```python
from build123d import *

# Parameters (mm, degrees)
CYLINDER002_R       = 0.3
CYLINDER002_DEPTH   = 10
CYLINDER001_R       = 0.3
CYLINDER001_DEPTH   = 10
CYLINDER_R          = 5.75
CYLINDER_DEPTH      = 6
CYLINDER_ROLL_ANGLE = 90
FILLET_R            = 2.2


with BuildPart() as pin002:
    # Cylinder002 → Cylinder002 (new body)
    with BuildSketch(Plane(origin=(2.5, 0, -3), x_dir=(1, 0, 0), z_dir=(0, 0, 1))):
        Circle(CYLINDER002_R)
    extrude(amount=CYLINDER002_DEPTH)


with BuildPart() as pin1:
    # Cylinder001 → Cylinder001 (new body)
    with BuildSketch(Plane(origin=(-2.5, 0, -3), x_dir=(1, 0, 0), z_dir=(0, 0, 1))):
        Circle(CYLINDER001_R)
    extrude(amount=CYLINDER001_DEPTH)


with BuildPart() as obj1:
    # Cylinder → Cylinder (new body)
    with BuildSketch(Plane.XY):
        Circle(CYLINDER_R)
    extrude(amount=CYLINDER_DEPTH)


with BuildPart() as obj1_1:
    # Cylinder roll: moved
    add(obj1.part.rotate(Axis((0, 0, 0), (1, 0, 0)), CYLINDER_ROLL_ANGLE))


with BuildPart() as obj1_2:
    # Cylinder placement: moved
    add(obj1_1.part.moved(Location((0, 3, 10.25))))

    # Fillet
    fillet_edges = [obj1_2.edges().sort_by_distance(p)[0] for p in [
        (-5.75, -3, 10.25),
        (-5.75, 3, 10.25),
    ]]
    fillet(fillet_edges, radius=FILLET_R)

    # Fusion: union pin002, pin1
    add(pin002.part)
    add(pin1.part)


solid = obj1_2.part
```
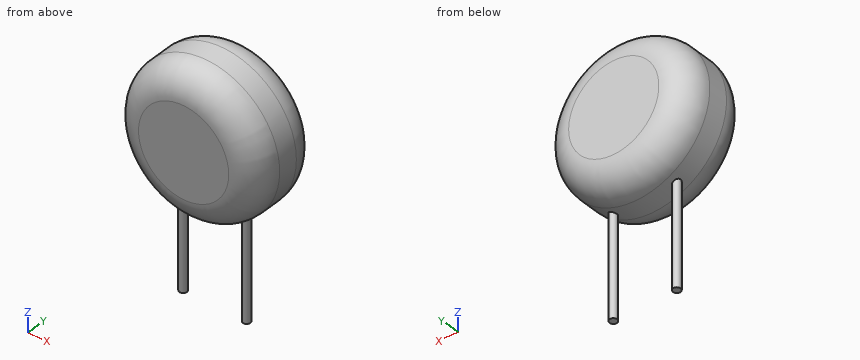
Read the model definition and answer for the solid it produces. Units are mm, in the model's axes. Coordinates: 2 decimals unless noted, no trailing zeros. Order: outer loops, then holes, each group sorted by start corner. A loop starts at its lowest first (then second) coordinate and runs counter-clockwise, first axis right, second up. Notation, with made-up numbers: (-5.75, 12) - (52.25, 12) arc R14 cw to (52.25, 31) - close; hole circle Ø3 at (-15, 41.25). An arc over 180 degrees is marked (long way). Answer as a JSON object with one key per item and string values. Group by question number.
Item 1: Section C-C (z = 3) is taken. Give the vertices of the cut face in (x, y), plus the area to 3 significant figures.
Item 2: Section A-A (x = 0) is taken. Give the vertices of the cut face in (y, z), plus the area to 3 significant figures.
Item 3: Section D-D (y = 0.5) is taken. Give the vertices of the cut face in (x, z).
Item 4: Consider probe 1 along Z at (x, y) = (-0.75, 0.25); probe 2 along Z at (x, y) = (-1.25, -1.75); probe 3 along Y at (x, z) = (0.25, 5). Determine where each line is inside the solid, lowest interval first. Write a range as from..to.
Item 5: Flat-ended cylindrical pins translate along their axes: P1, Ø1, axis at y = -2, z = 5.5, coming from the -X side; P2, Ø3, axis at x = 2, z = 0, coming from the +Y side. Find the tip coordinate at first contact, or state that the pin passes through.
Item 6: Section B-B (z = 10.25) is taken. Give the vertices of the cut face in (x, y).
Results are:
{
 "1": {"outline": "circle Ø0.6 at (-2.5, 0); circle Ø0.6 at (2.5, 0)", "area": "0.565 mm^2"},
 "2": {"outline": "(-3, 6.7) arc R2.2 ccw to (-0.8, 4.5) - (0.8, 4.5) arc R2.2 ccw to (3, 6.7) - (3, 13.8) arc R2.2 ccw to (0.8, 16) - (-0.8, 16) arc R2.2 ccw to (-3, 13.8) - close", "area": "64.8 mm^2"},
 "3": {"outline": "circle Ø11.5 at (0, 10.25)"},
 "4": {"probe 1": "z = 4.55..15.95", "probe 2": "z = 4.86..15.64", "probe 3": "y = -2.19..2.19"},
 "5": {"P1": "stops at x = -3.46", "P2": "stops at y = 0.3"},
 "6": {"outline": "(-5.75, -0.8) arc R2.2 ccw to (-3.55, -3) - (3.55, -3) arc R2.2 ccw to (5.75, -0.8) - (5.75, 0.8) arc R2.2 ccw to (3.55, 3) - (-3.55, 3) arc R2.2 ccw to (-5.75, 0.8) - close"}
}
